Here's how the part is built. I have some questions about the finished solid (model axes, mm). Round coordinates to 2 decimals unless told otherwise and drop trailing zeros. Write each loop counter-clockwise with the first axis right and the second up, starting at its lowest first coordinate (ties: lowest second). Pieces come first, ordered by that corner, then holes. Notation, with made-up numbers: (44, -6.75) - (87, -6.75) arc R12 cw to (87, 14.25) - close; hole circle Ø2 at (7, -1.5). An arc over 180 degrees is marked (long way). Use one line per item in the form item = value. Start each with the question number.
1. Will this pin go through, and if not, where does the flat tip stop? pin 1 (3 mm diameter, centred on x = 72.91, y = -3.97, fed in from +Z).
2. I want a section at A-A, the plane x = 88. List the corners of the cut face in (y, z) for me (3 decimals), plus the area to 3 significant figures.
3. I want a section at B-B, the plane y = -47. List the corners of the cut face in (x, z) for me (3 decimals).
4. I want a section at D-D, the plane y = -16.5. List the corners of the cut face in (x, z) for me (3 decimals), plus the area to 3 significant figures.
5. If I drill on line 1 along X through (y, z) = (-61, 1.6) (3 decimals); line 2 along X through (y, z) = (-25, 0.3) (3 decimals); line 3 along Y through (x, z) = (7, 1.05) (3 decimals), over which ranges is the centre line in solid material (lowest first)?
6. I want a section at C-C, the plane x = 50.5. List the corners of the cut face in (y, z) for me (3 decimals), plus the area to 3 significant figures.
```python
from build123d import *

# Parameters (mm, degrees)
F0_W     = 94.1376832
F0_H     = 76.2
F0_W_2   = 11.5876832
F0_H_2   = 24
F0_W_3   = 28.6999934
F0_H_3   = 28.6999934
F1_DEPTH = 3.175
F2_R     = 1.7272
F3_DEPTH = 3.175


with BuildPart() as f1:
    # F0 (on Top) → F1 (new body)
    with BuildSketch(Plane.XY):
        with Locations((47.0688416, -38.1)):
            Rectangle(F0_W, F0_H)
        with Locations((8.9688416, -61.025)):
            Rectangle(F0_W_2, F0_H_2, mode=Mode.SUBTRACT)
        with Locations((85.1688416, -61.025)):
            Rectangle(F0_W_2, F0_H_2, mode=Mode.SUBTRACT)
        with Locations((47.0688416, -38.1)):
            Rectangle(F0_W_3, F0_H_3, mode=Mode.SUBTRACT)
        with Locations((8.9688416, -15.175)):
            Rectangle(F0_W_2, F0_H_2, mode=Mode.SUBTRACT)
        with Locations((85.1688416, -15.175)):
            Rectangle(F0_W_2, F0_H_2, mode=Mode.SUBTRACT)
    extrude(amount=F1_DEPTH)

    # F2 (on face) → F3 (cut, through all)
    with BuildSketch(Plane.XY.offset(3.175)):
        with Locations((21.231352, -3.96875)):
            Circle(F2_R)
        with Locations((72.9063312, -3.96875)):
            Circle(F2_R)
        with Locations((72.9063312, -72.23125)):
            Circle(F2_R)
        with Locations((21.231352, -72.23125)):
            Circle(F2_R)
    extrude(amount=-F3_DEPTH, mode=Mode.SUBTRACT)


solid = f1.part
```
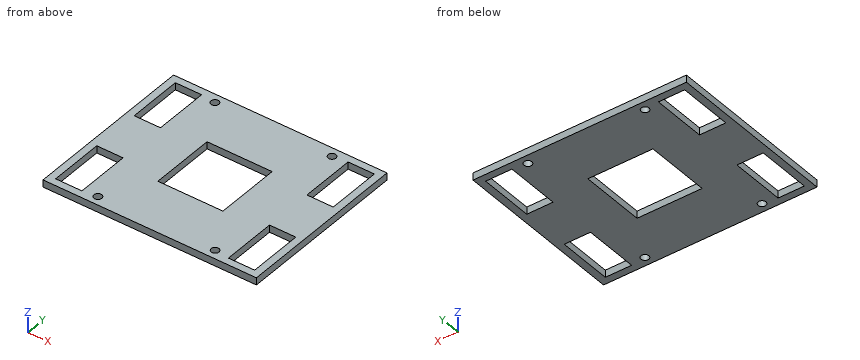
Model answer:
q1.pin_1 = through
q2.outline = (-76.2, 0) - (-73.025, 0) - (-73.025, 3.175) - (-76.2, 3.175) - close; (-49.025, 0) - (-27.175, 0) - (-27.175, 3.175) - (-49.025, 3.175) - close; (-3.175, 0) - (0, 0) - (0, 3.175) - (-3.175, 3.175) - close
q2.area = 89.5 mm2
q3.outline = (0, 0) - (32.719, 0) - (32.719, 3.175) - (0, 3.175) - close; (61.419, 0) - (94.138, 0) - (94.138, 3.175) - (61.419, 3.175) - close
q4.outline = (0, 0) - (3.175, 0) - (3.175, 3.175) - (0, 3.175) - close; (14.763, 0) - (79.375, 0) - (79.375, 3.175) - (14.763, 3.175) - close; (90.963, 0) - (94.138, 0) - (94.138, 3.175) - (90.963, 3.175) - close
q4.area = 225 mm2
q5.line_1 = 0 to 3.175, 14.763 to 79.375, 90.963 to 94.138
q5.line_2 = 0 to 3.175, 14.763 to 32.719, 61.419 to 79.375, 90.963 to 94.138
q5.line_3 = -76.2 to -73.025, -49.025 to -27.175, -3.175 to 0
q6.outline = (-76.2, 0) - (-52.45, 0) - (-52.45, 3.175) - (-76.2, 3.175) - close; (-23.75, 0) - (0, 0) - (0, 3.175) - (-23.75, 3.175) - close
q6.area = 151 mm2
